Autodesk Inventor part; units mm, degrees
ref_plane "Work Plane5" through (-94, 0, 0) normal (-0.7071, 0, -0.7071) x (0, 1, 0)
ref_plane "Work Plane6" through (0, -10, 0) normal (0, -1, 0) x (1, 0, 0)
ref_plane "YZ Plane" through (0, 0, 0) normal (1, 0, 0) x (0, 1, 0)
sketch "Sketch1" plane through (0, 0, 0) normal (0, 1, 0) x (-1, 0, 0)
  line L0 (0, 0) -> (94, 0)
  line L1 (94, 0) -> (94, -94)
  line L2 (94, -94) -> (0, -94)
  line L3 (0, -94) -> (0, 0)
  dimension "d0" = 94
  dimension "d1" = 94
extrude "Extrusion1" add sketch "Sketch1" along normal blind 4.5
sketch "Sketch2" plane through (0, 4.5, 0) normal (0, 1, 0) x (1, 0, 0)
  circle A0 centre (-47, 47) radius 12.5
  point P0 (0, 0)
  dimension "d4" = 25
  dimension "d5" = 47
  dimension "d6" = 47
extrude "Extrusion2" cut sketch "Sketch2" against normal blind 4.5
ref_plane "Work Plane3" through (-54.5, 0, 0) normal (1, 0, 0) x (0, 0, -1)
sketch "Sketch4" plane through (0, 4.5, 0) normal (0, 1, 0) x (1, 0, 0)
  line L0 (0, 94) -> (-94, 94)
  line L1 (-94, 94) -> (-94, 0)
  line L2 (0, 94) -> (-94, 0)
  circle A0 centre (-27.201, 66.799) radius 3
  line L3 (-94, 94) -> (0, 0)
  circle A1 centre (-66.799, 27.201) radius 3
  circle A2 centre (-55, 23) radius 2
  circle A3 centre (-39, 23) radius 2
  circle A4 centre (-55, 7) radius 2
  circle A5 centre (-39, 7) radius 2
  line L4 (-94, 0) -> (0, 0)
  line L5 (-47, 94) -> (-47, 0)
  line L6 (0, 0) -> (0, 94)
  circle A6 centre (-47, 47) radius 12.5
  point P0 (-47, 47)
  dimension "d21" = 6
  dimension "d25" = 4
  dimension "d26" = 4
  dimension "d27" = 4
  dimension "d28" = 4
  dimension "d29" = 16
  dimension "d30" = 16
  dimension "d31" = 16
  dimension "d32" = 16
  dimension "d33" = 7
  dimension "d34" = 39
  dimension "d35" = 7
  dimension "d36" = 39
  dimension "d66" = 28
extrude "Extrusion4" cut sketch "Sketch4" against normal blind 10 contours A0 L2 | L2 A0 | A1 L2 | L2 A1
extrude "Extrusion5" cut sketch "Sketch4" against normal blind 10 contours A2 | A3 | A4 | A5
sketch "Sketch5" plane through (0, 4.5, 0) normal (0, 1, 0) x (1, 0, 0)
  circle A0 centre (-47, 47) radius 12.5
  line L0 (-59.5, 47) -> (-59.5, 0)
  line L1 (-59.5, 47) -> (0, 47)
  line L2 (0, 0) -> (0, 94)
  circle A1 centre (-47, 47) radius 12.5
  line L3 (-94, 0) -> (0, 0)
  line L4 (-59.5, 0) -> (0, 0)
  line L5 (0, 0) -> (0, 47)
  circle A2 centre (-55, 7) radius 2
  circle A3 centre (-55, 7) radius 2
  circle A4 centre (-55, 23) radius 2
  circle A5 centre (-55, 23) radius 2
  circle A6 centre (-39, 23) radius 2
  circle A7 centre (-39, 23) radius 2
  circle A8 centre (-39, 7) radius 2
  circle A9 centre (-39, 7) radius 2
  point P0 (-34.5, 47)
extrude "Extrusion6" add sketch "Sketch5" along normal blind 15 contours L1 L2 L3 L0 A0
ref_plane "Work Plane5" through (-94, 0, 0) normal (-0.7071, 0, -0.7071) x (0, 1, 0)
ref_plane "Work Plane6" through (0, -10, 0) normal (0, -1, 0) x (1, 0, 0)
properties part number "box cover" material "Wood (Birch)"
The listing builds one solid part. Answer for the finished solid, in the listing's coordinates (mm). A direction names the side the tool comes from. Coordinates: 2 decimals unless noted, no trailing zeros. Write each loop counter-clockwise with the first axis right and the second up, starting at its lowest first coordinate (ties: lowest second). Pieces come first, ordered by that corner, then holes. Notation, with made-up numbers: M 30.25,62.5 L 83.25,62.5 A22 cw 83.25,91.5 Z; hole C -19,61 d7. An arc over 180 degrees is marked long. Write each question's results on one line, items separated by ' | '.
Item 1: The part is cut by section B-B on x = -47. Determine the outline of the cut face in (y, z).
Answer below:
outline: M 0,-94 L 4.5,-94 L 4.5,-59.5 L 0,-59.5 Z; M 0,-34.5 L 19.5,-34.5 L 19.5,0 L 0,0 Z
Item 2: The part is cut by section D-D on z = -23. Determine the outline of the cut face in (x, y).
Answer below:
outline: M -94,0 L -57,0 L -57,19.5 L -59.5,19.5 L -59.5,4.5 L -94,4.5 Z; M -53,0 L -41,0 L -41,19.5 L -53,19.5 Z; M -37,0 L 0,0 L 0,19.5 L -37,19.5 Z
Item 3: Which of the six approach directions +Z, -Z, +X, -X, +Y, -Y give full straight-line access (tool end or side, diameter ignored) to faces 4 (the face through (-36, 0, -36)), 5 (the face through (-57, 4.5, -57)), 6 (the face through (-41, 10, -7)), 7 (the face through (-17, 12, -47)), 8 (the face through (-59.5, 12, -24))?
Answer below:
face 4: +Z, -Z, +X, -X, -Y | face 5: -Z, -X, +Y | face 6: +Y, -Y | face 7: -Z, +X, -X, +Y | face 8: +Z, -Z, -X, +Y
Item 4: Given P1, Ø1.5, axis at x = -33, y = 10.5, coming from the -Z side; P2, Ø3.5, axis at x = -66.799, z = -27.201, coming from the -Y side; P3, Ø6, axis at x = -63, z = -22.5, coming from the +Y side, each flat-ended and moving along its own axis, determine where each tip first touches the part or whether it passes through.
Answer below:
P1: z = -47 | P2: through | P3: y = 4.5
Item 5: The part is cut by section C-C on y = 13. Determine the outline of the cut face in (x, z).
Answer below:
outline: M -59.5,-47 A12.5 cw -34.5,-47 L 0,-47 L 0,0 L -59.5,0 Z; hole C -55,-23 d4; hole C -55,-7 d4; hole C -39,-23 d4; hole C -39,-7 d4
Item 6: The part is cut by section A-A on z = -50.5. Determine the outline of the cut face in (x, y), and give its area (3 significant figures).
Answer below:
outline: M -94,0 L -59,0 L -59,4.5 L -94,4.5 Z; M -35,0 L 0,0 L 0,4.5 L -35,4.5 Z | area: 315 mm2
Item 7: Consider probe 1 along X at (y, z) = (6.75, -23); probe 2 along Z at (x, y) = (-55, 11.75); probe 3 along X at (y, z) = (15.25, -13). Determine where each line is inside the solid, lowest interval first. Write a range as [from, to].
Answer below:
probe 1: [-59.5, -57], [-53, -41], [-37, 0] | probe 2: [-37.4, -25], [-21, -9], [-5, 0] | probe 3: [-59.5, 0]
Item 8: For a pull along Z with two mould halves and no side action, classify faces 1 (the face through (0, 7, -27)), 2 (the face through (-48, 2, -94)), 3 (the face through (-48.627, 7.447, -34.606)) as released by +Z, released by -Z, zero draft, split by the parting line, or undercut.
Answer below:
face 1: zero draft | face 2: released by -Z | face 3: undercut
